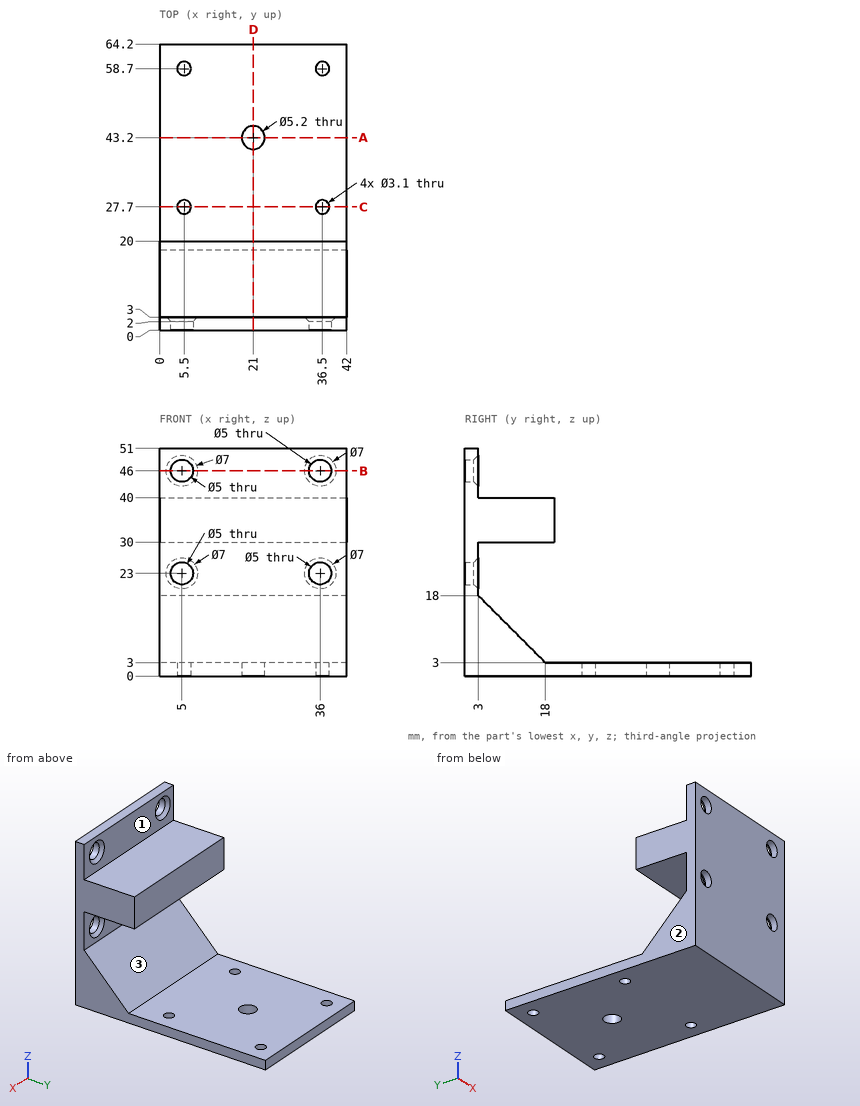
Here's the drawing with two shaded views (mm, measured from the low corner). I have some questions. A direction names the side the tool comes from. Coordinates: 2 decimals unless noted, no trailing zeros. Loops run counter-clockwise (first coordinate to the right, second up) from the corner with the lowest first, then second, coordinate; pieces in that order, holes last. Notation, with made-up numbers: (82.5, 45.5) -> (126.5, 45.5) arc R20 cw to (126.5, 79.5) -> close; hole circle Ø1 at (-16, 13). An arc over 180 degrees is marked (long way). Answer as a JSON object with one key per item and string values.
1) Imagine slicing it at C-C (y = 27.7). Please give me the cut outline in (x, z), then the cut area to 3 significant figures.
Results:
{"outline": "(0, 0) -> (3.95, 0) -> (3.95, 3) -> (0, 3) -> close; (7.05, 0) -> (34.95, 0) -> (34.95, 3) -> (7.05, 3) -> close; (38.05, 0) -> (42, 0) -> (42, 3) -> (38.05, 3) -> close", "area": "107 mm^2"}
2) Imagine slicing it at A-A (y = 43.2). Please give me the cut outline in (x, z), then the cut area to 3 significant figures.
Results:
{"outline": "(0, 0) -> (18.4, 0) -> (18.4, 3) -> (0, 3) -> close; (23.6, 0) -> (42, 0) -> (42, 3) -> (23.6, 3) -> close", "area": "110 mm^2"}
3) For the marked faces 1, 2 and 3, which set-ups out of +Z, -Z, +X, -X, +Y, -Y let a thin tool reach every point of the face, with its end or its side?
Results:
{"face 1": "+Z, +X, -X, +Y", "face 2": "+Z, -Z, -X, +Y, -Y", "face 3": "+X, -X, +Y"}
4) If I drill on line 1 (Z direction, x = 36, y = 0.9); line 2 (Y direction, x = 36.5, z = 1.9); line 3 (X direction, y = 0.7, z = 23), over which ranges is the centre line in solid material (lowest first)?
Results:
{"line 1": "z = 0 to 20.5, 25.5 to 43.5, 48.5 to 51", "line 2": "y = 0 to 26.15, 29.25 to 57.15, 60.25 to 64.2", "line 3": "x = 0 to 2.5, 7.5 to 33.5, 38.5 to 42"}
5) For P1, Ø5, axis at x = 23.5, y = 10.5, coming from the -Z side; P2, Ø1.5, axis at x = 9, y = 10.5, coming from the +Z side; P3, Ø5.5, axis at x = 17, z = 48, coming from the +Y side; P4, Ø3, axis at x = 13.5, z = 35.5, coming from the +Y side, each with a flat end and sliding along its axis, tell me the tip position at first contact or that it passes through.
Results:
{"P1": "stops at z = 0", "P2": "stops at z = 40", "P3": "stops at y = 3", "P4": "stops at y = 20"}
6) Imagine slicing it at D-D (x = 21). Please give me the cut outline in (y, z), then the cut area to 4 significant figures.
Results:
{"outline": "(0, 0) -> (40.6, 0) -> (40.6, 3) -> (18, 3) -> (3, 18) -> (3, 30) -> (20, 30) -> (20, 40) -> (3, 40) -> (3, 51) -> (0, 51) -> close; (45.8, 0) -> (64.2, 0) -> (64.2, 3) -> (45.8, 3) -> close", "area": "603.5 mm^2"}
7) Imagine slicing it at B-B (z = 46). Please give me the cut outline in (x, y).
Results:
{"outline": "(0, 0) -> (2.5, 0) -> (2.5, 2) -> (1.5, 3) -> (0, 3) -> close; (7.5, 0) -> (33.5, 0) -> (33.5, 2) -> (32.5, 3) -> (8.5, 3) -> (7.5, 2) -> close; (38.5, 0) -> (42, 0) -> (42, 3) -> (39.5, 3) -> (38.5, 2) -> close"}
